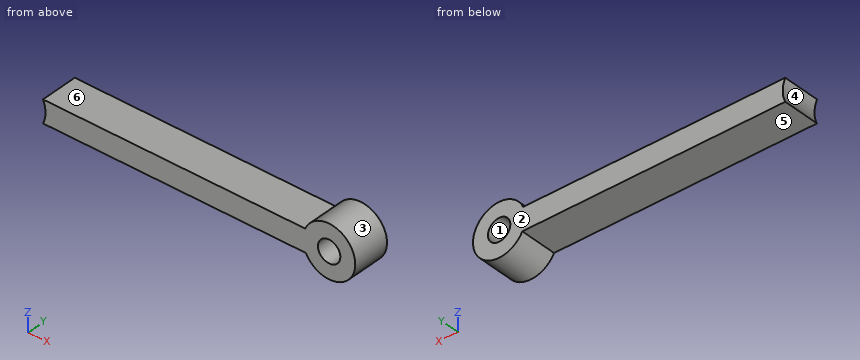
from build123d import *

# Parameters (mm, degrees)
BOSS_EXTRU_2_DEPTH      = 100
ESQUISSE5_R             = 30
ENL_V_MAT_EXTRU_4_DEPTH = 101
ESQUISSE6_R             = 70
ENL_V_MAT_EXTRU_5_DEPTH = 101


with BuildPart() as part:
    # Esquisse1 → Boss.-Extru.2 (new body)
    with BuildSketch(Plane(origin=(0, 0, 0), x_dir=(1, 0, 0), z_dir=(0, 1, 0))):
        with BuildLine():
            Line((379.401849177, 30.095541494), (-327.704932009, 30.095541494))
            Line((-327.704932009, 30.095541494), (-327.704932009, -30.095541494))
            Line((-327.704932009, -30.095541494), (377.209706533, -30.095541494))
            ThreePointArc((377.209706533, -30.095541494), (511.408174051, -4.847552565), (379.401849177, 30.095541494))
        make_face()
    extrude(amount=BOSS_EXTRU_2_DEPTH)

    # Esquisse5 → Enlèv. mat.-Extru.4 (cut, through all)
    with BuildSketch(Plane(origin=(0, 100, 0), x_dir=(1, 0, 0), z_dir=(0, 1, 0))):
        with Locations((441.45455179, -2.299860933)):
            Circle(ESQUISSE5_R)
    extrude(amount=-ENL_V_MAT_EXTRU_4_DEPTH, mode=Mode.SUBTRACT)

    # Esquisse6 → Enlèv. mat.-Extru.5 (cut, through all)
    with BuildSketch(Plane(origin=(0, 100, 0), x_dir=(1, 0, 0), z_dir=(0, 1, 0))):
        with Locations((-387.729757148, 0)):
            Circle(ESQUISSE6_R)
    extrude(amount=-ENL_V_MAT_EXTRU_5_DEPTH, mode=Mode.SUBTRACT)


solid = part.part
The listing builds one solid part. Answer for the finished solid, in the listing's coordinates (mm). Face numbers are marked on the shaded views. A direction names the side the tool comes from. Coordinates: 2 decimals unless noted, no trailing zeros. Write each loop counter-clockwise with the first axis right and the second up, starting at its lowest first coordinate (ties: lowest second). Pieces come first, ordered by that corner, then holes. Notation, with made-up numbers: (-1.75, -22) - (56.25, -22) arc R8 ccw to (56.25, -17) - close; hole circle Ø7 at (-14, -40). An arc over 180 degrees is marked (long way). Answer as CSV lines item,"result".
1. Given P1, Ø2, axis at y = 61.5, z = -49.5, coming from the -X side; P2, Ø4, axis at x = 13, y = 66, coming from the +Z side; P3, Ø12, axis at x = 109.5, y = 65, coming from the -Z side; P4, Ø5, axis at y = 63.5, z = -29.5, coming from the -X side, each flat-ended and moving along its own axis, determine where each tip first touches the part or whether it passes through.
Computed values:
P1,"stops at x = 393.29"
P2,"stops at z = 30.1"
P3,"stops at z = -30.1"
P4,"stops at x = -324.53"
2. Determine the mould class of the marked faces 1, 2 and 3 for opening direction Z: +Z half, -Z half, draft (parallel to the pull), parting line (faces both ways), or undercut.
Computed values:
face 1,"undercut"
face 2,"draft"
face 3,"parting line"
3. Find section D-D (z = 63). Give the vertices of the cut face in (x, y).
Computed values:
outline,"(406.59, 0) - (476.32, 0) - (476.32, 100) - (406.59, 100) - close"
4. Find section C-C (x = -133.5). Give the vertices of the cut face in (y, z).
Computed values:
outline,"(0, -30.1) - (100, -30.1) - (100, 30.1) - (0, 30.1) - close"
5. Find section A-A (z = -16.5). Give the vertices of the cut face in (x, y).
Computed values:
outline,"(-319.7, 0) - (418.08, 0) - (418.08, 100) - (-319.7, 100) - close; (464.83, 0) - (508.88, 0) - (508.88, 100) - (464.83, 100) - close"
6. Find section B-B (y = 56.5). Give the vertices of the cut face in (x, z).
Computed values:
outline,"(-324.53, -30.1) - (379.4, -30.1) arc R70 ccw (long way) to (377.21, 30.1) - (-324.53, 30.1) arc R70 cw to start; hole circle Ø60 at (441.45, 2.3)"
7. A tool of negligible diameter and unlimited length cuts with its end or side. For the marked faces 4, 5 and 6, from which of +Z, -Z, +X, -X, +Y, -Y can it reach the whole face along a straight path? Write none if from no direction.
Computed values:
face 4,"-X, +Y, -Y"
face 5,"-Z, -X, +Y, -Y"
face 6,"+Z, -X, +Y, -Y"
8. Straight lines are drawn through the part: line 1 (X direction, y = 50, z = -0.5); line 2 (Z direction, x = 217.5, y = 70.5); line 3 (X direction, y = 89.5, z = 22). For each, find the intervals that lie inside material, in ascending order. Write a range as [from, to].
Computed values:
line 1,"x = [-317.73, 411.59], [471.32, 511.4]"
line 2,"z = [-30.1, 30.1]"
line 3,"x = [-321.28, 418.83], [464.08, 508.63]"
